Check sheet for the modelled part. Datum: model origin and axes. Units: mm. Face numbers are marked on the shaded views. A direction names the side the tool comes from. Give positions to 0.01 mm unless a question says otherwise; leave off trailing zeros. Order: outer loops, then holes, each group sorted by start corner. A loop starts at its lowest first (then second) coordinate and runs counter-clockwise, first axis right, second up. Notation, with made-up numbers: (-10.5, -18.5) - (4.5, -18.5) arc R14 ccw to (4.5, -14.5) - close; hole circle Ø3 at (-28, 56). An arc over 180 degrees is marked (long way). Answer in a Markdown table with one row per item.
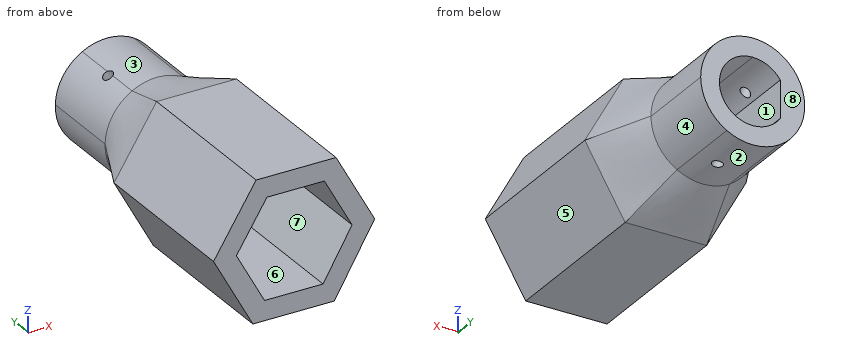
Autodesk Inventor part; units mm, degrees
ref_plane "YZ Plane" through (0, 0, 0) normal (1, 0, 0) x (0, 1, 0)
ref_plane "XZ Plane" through (0, 0, 0) normal (0, 1, 0) x (-1, 0, 0)
ref_plane "XY Plane" through (0, 0, 0) normal (0, 0, 1) x (1, 0, 0)
sketch "Sketch1" plane through (0, 0, 0) normal (0, 1, 0) x (-1, 0, 0)
  line L0 (3.0315, -4.7903) -> (-2.5932, -4.7903)
  line L1 (-2.5932, -4.7903) -> (-5.3821, -0.0266)
  line L2 (-5.3821, -0.0266) -> (-2.721, 4.8097)
  line L3 (-2.721, 4.8097) -> (2.7981, 4.8097)
  line L4 (2.7981, 4.8097) -> (5.7396, 0.1397)
  line L5 (5.7396, 0.1397) -> (3.0315, -4.7903)
  line L6 (-7.5579, -0.0555) -> (-3.6782, -6.6826)
  line L7 (-3.6782, -6.6826) -> (4.1511, -6.6826)
  line L8 (4.1511, -6.6826) -> (7.9347, 0.2053)
  line L9 (7.9347, 0.2053) -> (3.8427, 6.7021)
  line L10 (3.8427, 6.7021) -> (-3.8397, 6.7021)
  line L11 (-3.8397, 6.7021) -> (-7.5579, -0.0555)
  line L12 (0.004, -1.2887) -> (0.004, -3.3542)
  dimension "d43" = 9.6
ref_plane "Work Plane1" through (0, 14.35, 0) normal (0, 1, 0) x (1, 0, 0)
sketch "Sketch3" plane through (0, 14.35, 0) normal (0, 1, 0) x (1, 0, 0)
  circle A0 centre (0, 0) radius 5
  dimension "d7" = 10
extrude "Extrusion3" add sketch "Sketch1" along normal blind 8
sketch "Sketch6" plane through (0, 8, 0) normal (0, 1, 0) x (1, 0, 0)
  line L0 (3.6782, 6.6826) -> (-4.1511, 6.6826)
  line L1 (-4.1511, 6.6826) -> (-7.9347, -0.2053)
  line L2 (-7.9347, -0.2053) -> (-3.8427, -6.7021)
  line L3 (-3.8427, -6.7021) -> (3.8397, -6.7021)
  line L4 (3.8397, -6.7021) -> (7.5579, 0.0555)
  line L5 (7.5579, 0.0555) -> (3.6782, 6.6826)
  line L6 (-3.0315, 4.7903) -> (2.5932, 4.7903)
  line L7 (2.5932, 4.7903) -> (5.3821, 0.0266)
  line L8 (5.3821, 0.0266) -> (2.721, -4.8097)
  line L9 (2.721, -4.8097) -> (-2.7981, -4.8097)
  line L10 (-2.7981, -4.8097) -> (-5.7396, -0.1397)
  line L11 (-5.7396, -0.1397) -> (-3.0315, 4.7903)
  point P0 (0, 0)
loft "Loft2" add profiles "Sketch3" section 1 edges at (-0.2365, 8, -6.6826) (-6.0429, 8, -3.2387) (-5.8887, 8, 3.4537) (-0.0015, 8, 6.7021) (5.6988, 8, 3.3233) (5.618, 8, -3.3691)
sketch "Sketch7" plane through (0, 14.35, 0) normal (0, 1, 0) x (0.9999645, 0, -0.0084267)
  arc A0 (2.5271, 4.3143) -> (-2.5271, 4.3143) centre (0, 0) ccw
  arc A1 (-2.5271, 4.3143) -> (-4.9992, -0.09) centre (0, 0) ccw
  arc A2 (-4.9992, -0.09) -> (-2.4442, -4.3618) centre (0, 0) ccw
  arc A3 (-2.4442, -4.3618) -> (2.5264, -4.3148) centre (0, 0) ccw
  arc A4 (2.5264, -4.3148) -> (5, -0.0063) centre (0, 0) ccw
  arc A5 (5, -0.0063) -> (2.5271, 4.3143) centre (0, 0) ccw
  point P0 (0, 0)
sketch "Sketch8" plane through (0, 0, 0) normal (0, -1, 0) x (1, 0, 0)
  line L0 (3.6782, -6.6826) -> (-4.1511, -6.6826)
  line L1 (7.5579, -0.0555) -> (3.6782, -6.6826)
  line L2 (3.8397, 6.7021) -> (7.5579, -0.0555)
  line L3 (-3.8427, 6.7021) -> (3.8397, 6.7021)
  line L4 (-7.9347, 0.2053) -> (-3.8427, 6.7021)
  line L5 (-4.1511, -6.6826) -> (-7.9347, 0.2053)
  line L6 (-3.0315, -4.7903) -> (2.5932, -4.7903)
  line L7 (-5.7396, 0.1397) -> (-3.0315, -4.7903)
  line L8 (-2.7981, 4.8097) -> (-5.7396, 0.1397)
  line L9 (2.721, 4.8097) -> (-2.7981, 4.8097)
  line L10 (5.3821, -0.0266) -> (2.721, 4.8097)
  line L11 (2.5932, -4.7903) -> (5.3821, -0.0266)
  point P0 (0, 0)
extrude "Extrusion4" add sketch "Sketch8" along normal blind 8
extrude "Extrusion5" add sketch "Sketch7" along normal blind 8
sketch "Sketch9" plane through (0, 22.35, 0) normal (0, 1, 0) x (1, 0, 0)
  point P0 (0, 0)
  point P1 (0, 0)
hole "Hole2" at (0, 22.35, 0) direction (0, -1, 0) diameter 6.4 end through all
ref_plane "Work Plane5" through (3.8397, 0, 6.7021) normal (-0.3395675, 0, 0.9405817) x (0, -1, 0)
sketch "Sketch10" plane through (3.8397, 0, 6.7021) normal (-0.3395675, 0, 0.9405817) x (0, -1, 0)
  point P0 (0, -5.8873)
  point P1 (-17.8788, -6.8855)
hole "Hole3" at (-2.6367, 17.8788, 4.3639) direction (0.3395675, 0, -0.9405817) diameter 1 end through all
sketch "Sketch11" plane through (0, 22.35, 0) normal (0, 1, 0) x (1, 0, 0)
  line L0 (-2.65, 7.87) -> (-2.65, -12.0471)
  circle A0 centre (0, 0) radius 3.2
  line L1 (3.05, 2.2452) -> (3.05, -2.0886)
  point P0 (0, 0)
  point P1 (-2.65, -1.7937)
  point P2 (-2.65, 1.7937)
  dimension "d52" = 3.05
  dimension "d53" = 5.7
extrude "Extrusion6" add sketch "Sketch11" against normal up to surface (14.35 mm away) contours L0 A0
properties part number "motorattacher"
(1) Cross-section at A-A, the plane y = 3.5. Record the cut outline in (x, z).
Geometry says:
| item | result |
|---|---|
| outline | (-7.93, 0.21) - (-4.15, -6.68) - (3.68, -6.68) - (7.56, -0.06) - (3.84, 6.7) - (-3.84, 6.7) - close; hole (-5.74, 0.14) - (-3.03, -4.79) - (2.59, -4.79) - (5.38, -0.03) - (2.72, 4.81) - (-2.8, 4.81) - close |
(2) Access from +Z, -Z, +X, -X, +Y, -Y to the whole of each face (thin tool, end or side, straight path). Record for the marked faces 1, 2, 3 and 4.
Geometry says:
| item | result |
|---|---|
| face 1 | +Y, -Y |
| face 2 | -Z, +Y |
| face 3 | +Z, +Y |
| face 4 | -Z, +X, +Y |
(3) Mould release check, pull along Z, two halves, no side actions. Record for the marked faces 5, 6, 7 and 8: pulls with the +Z half, pulls with the -Z half, needs draft (parallel to the pull), parting line crosses it, or undercut.
Geometry says:
| item | result |
|---|---|
| face 5 | pulls with the -Z half |
| face 6 | undercut |
| face 7 | undercut |
| face 8 | needs draft |
(4) Gauge pin test, flat ends, axial feed: P1, Ø2, axis at y = 15.5, z = 1, coming from the +X side; P2, Ø6, axis at y = 14.5, z = -2.5, coming from the +X side; P3, Ø1, axis at y = 9, z = -3, coming from the -X side. Record the tip position at first contact, or that the pin passes through.
Geometry says:
| item | result |
|---|---|
| P1 | x = 5 |
| P2 | x = 5.72 |
| P3 | x = -6.16 |
(5) Thickness scan on L1, parallel to X at y = 19.75, z = 0; L2, parallel to Z at x = -1.5, y = -2; L3, parallel to Y at x = 3.75, z = -2.5. Record the ranges inside material, lowest first.
Geometry says:
| item | result |
|---|---|
| L1 | -5 to -2.65, 3.2 to 5 |
| L2 | -6.68 to -4.79, 4.81 to 6.7 |
| L3 | 8 to 22.35 |
